The model under review builds one solid part; all positions refer to its coordinate system, in mm. Coordinates: 2 decimals unless noted, no trailing zeros. Write each loop counter-clockwise with the first axis right and the second up, starting at its lowest first coordinate (ties: lowest second). Pieces come first, ordered by that corner, then holes.
1) For line 1 (Z direction, x = -21.47, y = 1.5); line 2 (X direction, y = 2.75, z = -19); line 3 (X direction, y = 1.7, z = -16.66), list the stretches that pass through material, from the lowest coordinate up.
2) Add section B-B, the plane x = 0.57. State the section outline as (y, z) points, then the cut area to 3 significant figures.
3) Add section C-C, the plane y = 1. State the section outline as (x, z) points, then the cut area to 3 significant figures.
4) Add section A-A, the plane z = -7.62. State the section outline as (x, y) points.
5) Add section D-D, the plane z = -16.66. State the section outline as (x, y) points, then the cut area to 3 significant figures.
6) Mouldability with a two-part tool opening along X and no side actions: class faces 1 (the flat face through (-31.66, 2, 0)), 2 (the cylindrical face through (14.658, 1.578, -12.057)), 3 (the flat face through (-7, 0, 7)), 4 (the cylindrical face through (30.23, 1.62, 31.35)) as released by +X, released by -X, zero draft, split by the parting line, or undercut.
from build123d import *

# Parameters (mm, degrees)
SKETCH1_W           = 63.32
SKETCH1_H           = 65.7
SKETCH1_R           = 14.77
SKETCH1_R_2         = 3.81
BOSS_EXTRUDE1_DEPTH = 3.2
SKETCH2_OUTSIDE_W   = 83.58
SKETCH2_OUTSIDE_H   = 85.96
CUT_EXTRUDE1_DEPTH  = 3.2


with BuildPart() as part:
    # Sketch1 → Boss-Extrude1 (new body)
    with BuildSketch(Plane(origin=(0, 0, 0), x_dir=(1, 0, 0), z_dir=(0, 1, 0))):
        Rectangle(SKETCH1_W, SKETCH1_H)
        with Locations((0.57, 7.62)):
            Circle(SKETCH1_R, mode=Mode.SUBTRACT)
        with Locations((-21.47, 16.66)):
            Circle(SKETCH1_R_2, mode=Mode.SUBTRACT)
        with Locations((22.365921653, -1.31988801)):
            Circle(SKETCH1_R_2, mode=Mode.SUBTRACT)
    extrude(amount=BOSS_EXTRUDE1_DEPTH)

    # Sketch2 outside → Cut-Extrude1 (cut)
    with BuildSketch(Plane(origin=(0, 3.2, 0), x_dir=(1, 0, 0), z_dir=(0, 1, 0))):
        Rectangle(SKETCH2_OUTSIDE_W, SKETCH2_OUTSIDE_H)
        with BuildLine():
            Line((26.66, -32.85), (-26.66, -32.85))
            ThreePointArc((-26.66, -32.85), (-30.195533906, -31.385533906), (-31.66, -27.85))
            Line((-31.66, -27.85), (-31.66, 27.85))
            ThreePointArc((-31.66, 27.85), (-30.195533906, 31.385533906), (-26.66, 32.85))
            Line((-26.66, 32.85), (26.66, 32.85))
            ThreePointArc((26.66, 32.85), (30.195533906, 31.385533906), (31.66, 27.85))
            Line((31.66, 27.85), (31.66, -27.85))
            ThreePointArc((31.66, -27.85), (30.195533906, -31.385533906), (26.66, -32.85))
        make_face(mode=Mode.SUBTRACT)
    extrude(amount=-CUT_EXTRUDE1_DEPTH, mode=Mode.SUBTRACT)


solid = part.part
Geometry results:
1. line 1: z = -32.85 to -20.47, -12.85 to 32.85
1. line 2: x = -31.66 to -24.48, -18.46 to -8.85, 9.99 to 31.66
1. line 3: x = -31.66 to -25.28, -17.66 to -11.11, 12.25 to 31.66
2. outline: (0, -32.85) - (3.2, -32.85) - (3.2, -22.39) - (0, -22.39) - close; (0, 7.15) - (3.2, 7.15) - (3.2, 32.85) - (0, 32.85) - close
2. area: 116 mm2
3. outline: (-31.66, -27.85) arc R5 ccw to (-26.66, -32.85) - (26.66, -32.85) arc R5 ccw to (31.66, -27.85) - (31.66, 27.85) arc R5 ccw to (26.66, 32.85) - (-26.66, 32.85) arc R5 ccw to (-31.66, 27.85) - close; hole circle Ø7.62 at (-21.47, -16.66); hole circle Ø29.54 at (0.57, -7.62); hole circle Ø7.62 at (22.37, 1.32)
3. area: 3,360 mm2
4. outline: (-31.66, 0) - (-14.2, 0) - (-14.2, 3.2) - (-31.66, 3.2) - close; (15.34, 0) - (31.66, 0) - (31.66, 3.2) - (15.34, 3.2) - close
5. outline: (-31.66, 0) - (-25.28, 0) - (-25.28, 3.2) - (-31.66, 3.2) - close; (-17.66, 0) - (-11.11, 0) - (-11.11, 3.2) - (-17.66, 3.2) - close; (12.25, 0) - (31.66, 0) - (31.66, 3.2) - (12.25, 3.2) - close
5. area: 103 mm2
6. face 1: released by -X
6. face 2: undercut
6. face 3: zero draft
6. face 4: released by +X
